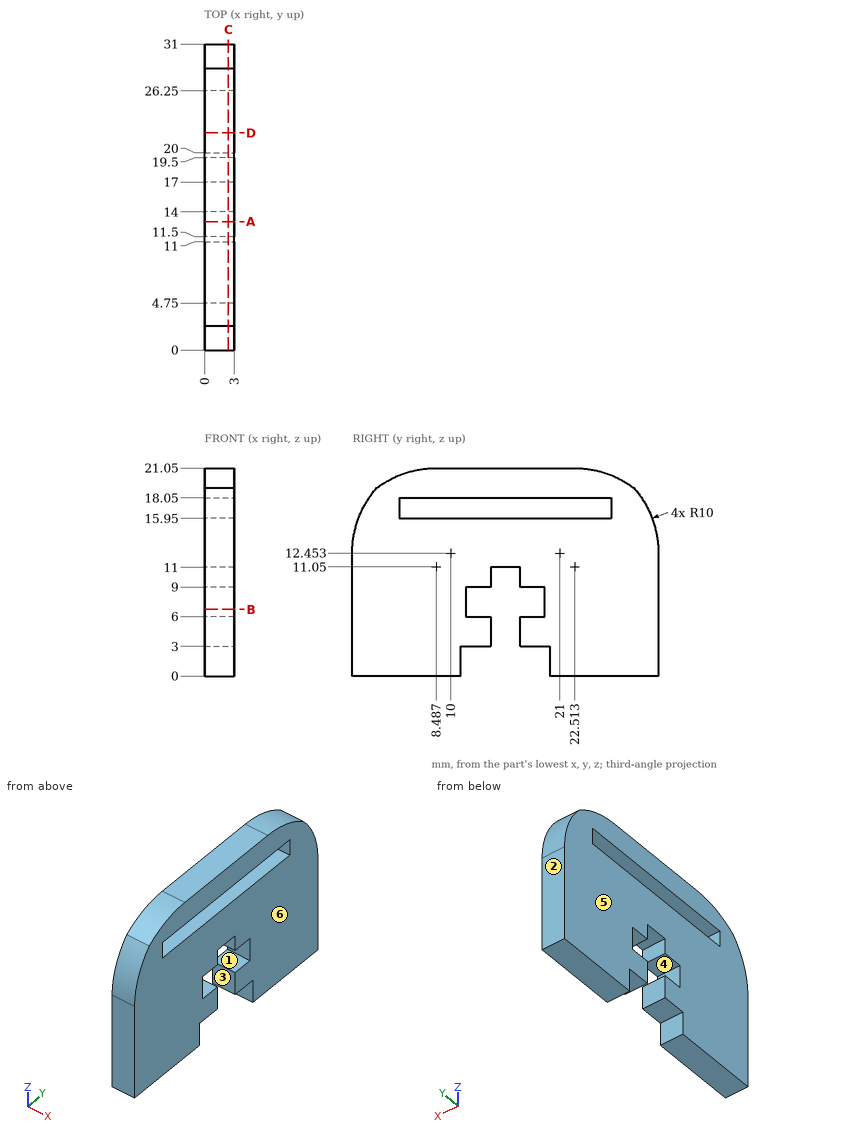
Drawing for the job (mm, zero at the part's lowest x, y, z). A direction names the side the tool comes from. Round coordinates to 2 decimals unless told otherwise and drop trailing zeros. Loops run counter-clockwise (first coordinate to the right, second up) from the corner with the lowest first, then second, coordinate; pieces in that order, holes last. Notation, with made-up numbers: M 83,36 L 108,36 A18 cw 108,57 Z; hole C -23.5,48 d8. An arc over 180 degrees is marked long. Use a Markdown table: item, result. Add a question column.
(1) Cut at A-A (y = 13). Give the cut face in (x, z).
(2) Which spindle directions (+Z, -Z, +X, -X, +Y, -Y) get a long thin tool onto all of the face, cutting with end or side? Do the marked faces 1, 2 and 3. Say none if no direction does.
(3) Flat gauge pins, fed straight in: pin 1 (1.1 mm diameter, centred on x = 2, z = 17, fed in from +Y); pin 2 (0.9 mm diameter, centred on x = 2, y = 15, fed in from -Z); pin 3 (0.9 mm diameter, centred on x = 2, y = 17, fed in from -Z). Where does each tip first touch, or does it go through?
(4) Pull direction X, two halves, no side cores. Call the marked faces 4, 5 and 6: +X half, -X half, draft (parallel to the pull), parting line (faces both ways), or undercut.
(5) Cut at B-B (z = 6.75). Give the cut face in (x, y), and give its area (3 significant figures).
(6) Cut at C-C (x = 2.4). Give the cut face in (y, z).
(7) Cut at D-D (y = 22). Give the cut face in (x, z).
(8) Drill centre lines: line 1 (Z direction, x = 0.75, y = 13); line 2 (Z direction, x = 0.8, y = 21); line 3 (Z direction, x = 2, y = 15.5). Where is each one in solid material? Low to high.
Geometry says:
| question | item | result |
|---|---|---|
| 1 | outline | M 0,3 L 3,3 L 3,6 L 0,6 Z; M 0,9 L 3,9 L 3,15.95 L 0,15.95 Z; M 0,18.05 L 3,18.05 L 3,21.05 L 0,21.05 Z |
| 2 | face 1 | +X, -X |
| 2 | face 2 | +Z, -Z, +X, -X, +Y |
| 2 | face 3 | -Z, +X, -X |
| 3 | pin 1 | stops at y = 30.17 |
| 3 | pin 2 | stops at z = 11 |
| 3 | pin 3 | stops at z = 3 |
| 4 | face 4 | draft |
| 4 | face 5 | -X half |
| 4 | face 6 | +X half |
| 5 | outline | M 0,0 L 3,0 L 3,11.5 L 0,11.5 Z; M 0,19.5 L 3,19.5 L 3,31 L 0,31 Z |
| 5 | area | 69.0 mm² |
| 6 | outline | M 0,0 L 11,0 L 11,3 L 14,3 L 14,6 L 11.5,6 L 11.5,9 L 14,9 L 14,11 L 17,11 L 17,9 L 19.5,9 L 19.5,6 L 17,6 L 17,3 L 20,3 L 20,0 L 31,0 L 31,12.45 A10 ccw 28.52,19.05 A10 ccw 22.51,21.05 L 8.49,21.05 A10 ccw 2.48,19.05 A10 ccw 0,12.45 Z; hole M 4.75,15.95 L 26.25,15.95 L 26.25,18.05 L 4.75,18.05 Z |
| 7 | outline | M 0,0 L 3,0 L 3,15.95 L 0,15.95 Z; M 0,18.05 L 3,18.05 L 3,21.05 L 0,21.05 Z |
| 8 | line 1 | z = 3 to 6, 9 to 15.95, 18.05 to 21.05 |
| 8 | line 2 | z = 0 to 15.95, 18.05 to 21.05 |
| 8 | line 3 | z = 11 to 15.95, 18.05 to 21.05 |
